Source: CAD feature listing. Evaluate the final solid. Frame: model axes, mm. Face numbers are marked on the shaded views. A direction names the side the tool comes from. Coordinates: 2 decimals unless noted, no trailing zeros. Order: outer loops, then holes, each group sorted by start corner. A loop starts at its lowest first (then second) coordinate and runs counter-clockwise, first axis right, second up.
Autodesk Inventor part; units mm, degrees
ref_plane "YZ Plane" through (0, 0, 0) normal (1, 0, 0) x (0, 1, 0)
ref_plane "XZ Plane" through (0, 0, 0) normal (0, 1, 0) x (-1, 0, 0)
ref_plane "XY Plane" through (0, 0, 0) normal (0, 0, 1) x (1, 0, 0)
sketch "Sketch1" plane through (0, 0, 0) normal (0, 0, 1) x (1, 0, 0)
  circle A0 centre (0, 0) radius 75
  dimension "d0" = 150
extrude "Extrusion1" add sketch "Sketch1" along normal mid plane 50
sketch "Sketch2" plane through (0, 0, 0) normal (0, 0, 1) x (1, 0, 0)
  circle A0 centre (0, 0) radius 50
  dimension "d3" = 100
extrude "Extrusion2" cut sketch "Sketch2" along normal mid plane 50
sketch "Sketch3" plane through (0, 0, 0) normal (0, 0, 1) x (1, 0, 0)
  circle A0 centre (0, 0) radius 25
  dimension "d6" = 50
extrude "Extrusion3" add sketch "Sketch3" along normal mid plane 50
sketch "Sketch10" plane through (0, 0, 25) normal (0, 0, 1) x (1, 0, 0)
  circle A0 centre (0, 0) radius 75
  circle A1 centre (0, 75) radius 12.5
  circle A2 centre (-44.0839, 60.6763) radius 12.5
  circle A3 centre (-71.3292, 23.1763) radius 12.5
  circle A4 centre (-71.3292, -23.1763) radius 12.5
  circle A5 centre (-44.0839, -60.6763) radius 12.5
  circle A6 centre (0, -75) radius 12.5
  circle A7 centre (44.0839, -60.6763) radius 12.5
  circle A8 centre (71.3292, -23.1763) radius 12.5
  circle A9 centre (71.3292, 23.1763) radius 12.5
  circle A10 centre (44.0839, 60.6763) radius 12.5
  dimension "d46" = 25
  dimension "d49" = 360
extrude "Extrusion9" cut sketch "Sketch10" against normal through all contours A9 A0 | A0 A9 | A8 A0 | A0 A8 | A10 A0 | A0 A10 | A7 A0 | A0 A7 | A1 A0 | A0 A1 | A6 A0 | A0 A6 | A2 A0 | A0 A2 | A5 A0 | A0 A5 | A3 A0 | A0 A3 | A4 A0 | A0 A4
sketch "Sketch11" plane through (0, 0, 0) normal (0, 0, 1) x (1, 0, 0)
  circle A0 centre (0, 0) radius 25 construction
  circle A1 centre (0, 0) radius 50 construction
  line L0 (0, 0) -> (50, 0) construction
  line L1 (-8.6824, 49.2404) -> (-14.3982, 20.4375)
  line L2 (8.6824, 49.2404) -> (14.3982, 20.4375)
  line L3 (-38.3022, -32.1394) -> (-10.5003, -22.6879)
  line L4 (-46.9846, -17.101) -> (-24.8985, 2.2504)
  line L5 (46.9846, -17.101) -> (24.8985, 2.2504)
  line L6 (38.3022, -32.1394) -> (10.5003, -22.6879)
  arc A2 (8.6824, 49.2404) -> (-8.6824, 49.2404) centre (0, 0) ccw
  arc A3 (-46.9846, -17.101) -> (-38.3022, -32.1394) centre (0, 0) ccw
  arc A4 (38.3022, -32.1394) -> (50, 0) centre (0, 0) ccw
  arc A5 (10.5003, -22.6879) -> (24.8985, 2.2504) centre (0, 0) ccw
  arc A6 (14.3982, 20.4375) -> (-14.3982, 20.4375) centre (0, 0) ccw
  arc A7 (-24.8985, 2.2504) -> (-10.5003, -22.6879) centre (0, 0) ccw
  dimension "d56" = 360
extrude "Extrusion10" add sketch "Sketch11" along normal mid plane 50
sketch "Sketch12" plane through (0, 0, 25) normal (0, 0, 1) x (1, 0, 0)
  circle A0 centre (0, 0) radius 15
  dimension "d60" = 30
extrude "Extrusion11" add sketch "Sketch12" along normal blind 20
sketch "Sketch13" plane through (0, 0, 45) normal (0, 0, 1) x (1, 0, 0)
  circle A0 centre (0, 0) radius 7.5
  dimension "d63" = 15
extrude "Extrusion12" cut sketch "Sketch13" against normal blind 20
properties part number "Guntas_Wheel_New"
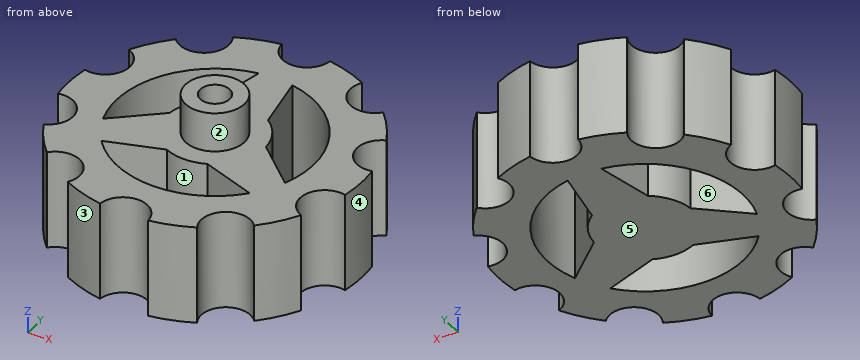
Q1. Set-up query: the marked faces 1, 2 and 3. Return all of +Z, -Z, +X, -X, +Y, -Y with unobstructed straight access to the full face (end or side cutting, diameter ignored); none if empty.
Solutions:
face 1: +Z, -Z
face 2: +Z
face 3: +Z, -Z, -X, -Y
Q2. Pin query (flat end, axial travel): P1, Ø12, axis at y = -13.5, z = 32.5, coming from the +X side; P2, Ø1.5, axis at x = -25.5, z = 9, coming from the -Y side; P3, Ø5, axis at x = 2, z = -7.5, coming from the -Y side; P4, Ø1, axis at x = 37.5, y = 53, coming from the +Z side. Return the tip coordinate at first contact, or that it passes through.
Solutions:
P1: stops at x = 12.99
P2: stops at y = -70.8
P3: stops at y = -63.34
P4: passes through
Q3. Section query A-A on x = 0. Output: boundary loops of the cut face in (y, z).
Solutions:
outline: (-62.5, -25) - (-50, -25) - (-50, 25) - (-62.5, 25) - close; (-25, -25) - (62.5, -25) - (62.5, 25) - (15, 25) - (15, 45) - (7.5, 45) - (7.5, 25) - (-7.5, 25) - (-7.5, 45) - (-15, 45) - (-15, 25) - (-25, 25) - close
Q4. Pull-direction query (Y, two-part tool) for the marked faces 4, 5 and 6; classes: pulls with the +Y half, pulls with the -Y half, needs draft (parallel to the pull), parting line crosses it, or undercut.
Solutions:
face 4: parting line crosses it
face 5: needs draft
face 6: undercut
Q5. Material intervals for line 1 along Y through (x, z) = (0, 39); line 2 along X through (y, z) = (45, -1); line 3 along Z through (x, y) = (21, -54), sorted ascending.
Solutions:
line 1: y = -15 to -7.5, 7.5 to 15
line 2: x = -60 to -21.79, -9.52 to 9.52, 21.79 to 60
line 3: z = -25 to 25
Q6. Section query B-B on y = 18.5. Output: boundary loops of the cut face in (x, z).
Solutions:
outline: (-59.74, -25) - (-46.45, -25) - (-46.45, 25) - (-59.74, 25) - close; (-16.82, -25) - (16.82, -25) - (16.82, 25) - (-16.82, 25) - close; (46.45, -25) - (59.74, -25) - (59.74, 25) - (46.45, 25) - close
Q7. Section query C-C on z = 3.5. Give the number of separate pieces and of enclosed holes in the cut face, plus the area to 3 significant figures.
Solutions:
separate pieces: 1
enclosed holes: 3
area: 11,200 mm2
Q8. Section query D-D on x = 17. Output: boundary loops of the cut face in (y, z), plus the area to 3 significant figures.
Solutions:
outline: (-73.05, -25) - (-47.02, -25) - (-47.02, 25) - (-73.05, 25) - close; (-24.9, -25) - (18.33, -25) - (18.33, 25) - (-24.9, 25) - close; (47.02, -25) - (73.05, -25) - (73.05, 25) - (47.02, 25) - close
area: 4,760 mm2
